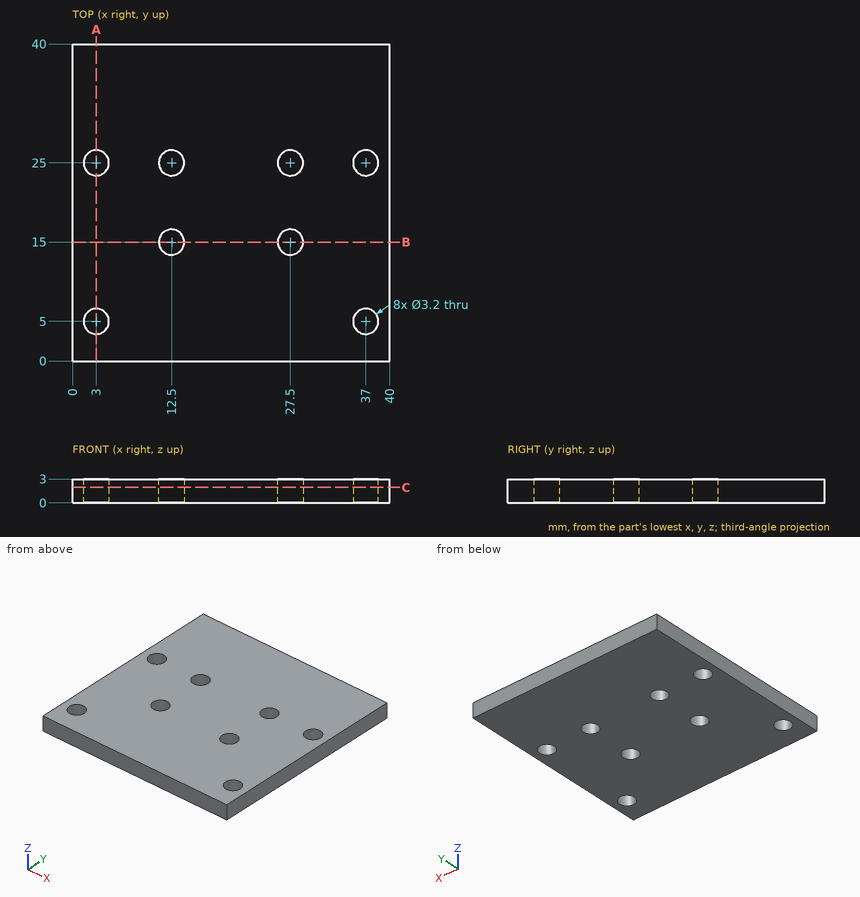
Answer from the drawing. Dimensions are ordinates in mm from the lowest x, y and z of the part. Coordinates: 2 decimals unless noted, no trailing zeros. Loops run counter-clockwise (first coordinate to the right, second up) from the corner with the lowest first, then second, coordinate; pieces in that order, holes last.
1) Flat-ended cylindrical pins translate along their axes: pin 1 (1 mm diameter, centred on y = 12, z = 0.5, fed in from -X); pin 2 (2.5 mm diameter, centred on x = 3, y = 25, fed in from -Z). Find the tip coordinate at first contact, or state that the pin passes through.
Results:
pin 1: stops at x = 0
pin 2: passes through
2) Section B-B (y = 15) is taken. Give the vertices of the cut face in (x, z), plus the area to 3 significant figures.
Results:
outline: (0, 0) - (10.9, 0) - (10.9, 3) - (0, 3) - close; (14.1, 0) - (25.9, 0) - (25.9, 3) - (14.1, 3) - close; (29.1, 0) - (40, 0) - (40, 3) - (29.1, 3) - close
area: 101 mm2
3) Section A-A (x = 3) is taken. Give the vertices of the cut face in (y, z).
Results:
outline: (0, 0) - (3.4, 0) - (3.4, 3) - (0, 3) - close; (6.6, 0) - (23.4, 0) - (23.4, 3) - (6.6, 3) - close; (26.6, 0) - (40, 0) - (40, 3) - (26.6, 3) - close
4) Section C-C (z = 1.95) is taken. Give the number of separate pieces and of enclosed holes in the cut face, plus the area to 3 significant figures.
Results:
separate pieces: 1
enclosed holes: 8
area: 1,540 mm2
5) Consider probe 1 along Y at (x, z) = (3, 1.6); probe 2 along Y at (x, z) = (12.5, 1.05); probe 3 along X at (y, z) = (15.5, 1.4). Determine where each line is inside the solid, lowest interval first.
Results:
probe 1: y = 0 to 3.4, 6.6 to 23.4, 26.6 to 40
probe 2: y = 0 to 13.4, 16.6 to 23.4, 26.6 to 40
probe 3: x = 0 to 10.98, 14.02 to 25.98, 29.02 to 40
